Part print with two shaded views. Sizes in mm from the minimum x, y, z corner. Round coordinates to 2 decimals unless told otherwise and drop trailing zeros. Loops run counter-clockwise (first coordinate to the right, second up) from the corner with the lowest first, then second, coordinate; pieces in that order, holes last. Notation, with made-up numbers: (2.5, -15) -> (16.5, -15) arc R22 ccw to (16.5, 9) -> close; hole circle Ø9 at (-40, -8). An arc over 180 degrees is marked (long way). Put each result on its own line as item: value. Start each with the question number.
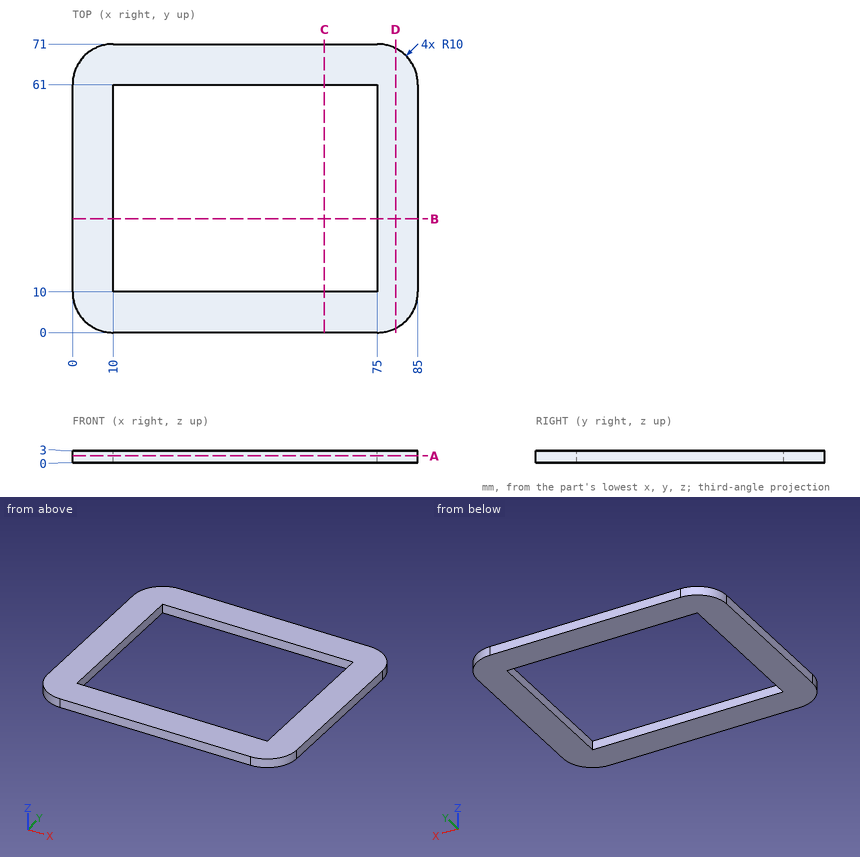
Item 1: Cut at D-D on x = 79.5. Write the cut outline in (y, z), then the cut area to 3 significant figures.
Item 2: Cut at B-B on y = 28. Write the cut outline in (x, z), then the cut area to 3 significant figures.
Item 3: Wall check: line 1 (X direction, y = 40, z = 0.65); line 2 (Y direction, x = 47.5, z = 2.8); line 3 (Y direction, x = 78.5, z = 2.5). Give the ranges that are in metal, low to high. Write a range as from..to.
Item 4: Cut at C-C on x = 62. Write the cut outline in (y, z).
Item 5: Cut at A-A on z = 1.7. Write the cut outline in (x, y), then the cut area to 3 significant figures.
Ans:
1. outline: (1.07, 0) -> (69.93, 0) -> (69.93, 3) -> (1.07, 3) -> close
1. area: 207 mm2
2. outline: (0, 0) -> (10, 0) -> (10, 3) -> (0, 3) -> close; (75, 0) -> (85, 0) -> (85, 3) -> (75, 3) -> close
2. area: 60.0 mm2
3. line 1: x = 0..10, 75..85
3. line 2: y = 0..10, 61..71
3. line 3: y = 0.63..70.37
4. outline: (0, 0) -> (10, 0) -> (10, 3) -> (0, 3) -> close; (61, 0) -> (71, 0) -> (71, 3) -> (61, 3) -> close
5. outline: (0, 10) arc R10 ccw to (10, 0) -> (75, 0) arc R10 ccw to (85, 10) -> (85, 61) arc R10 ccw to (75, 71) -> (10, 71) arc R10 ccw to (0, 61) -> close; hole (10, 10) -> (75, 10) -> (75, 61) -> (10, 61) -> close
5. area: 2,630 mm2
